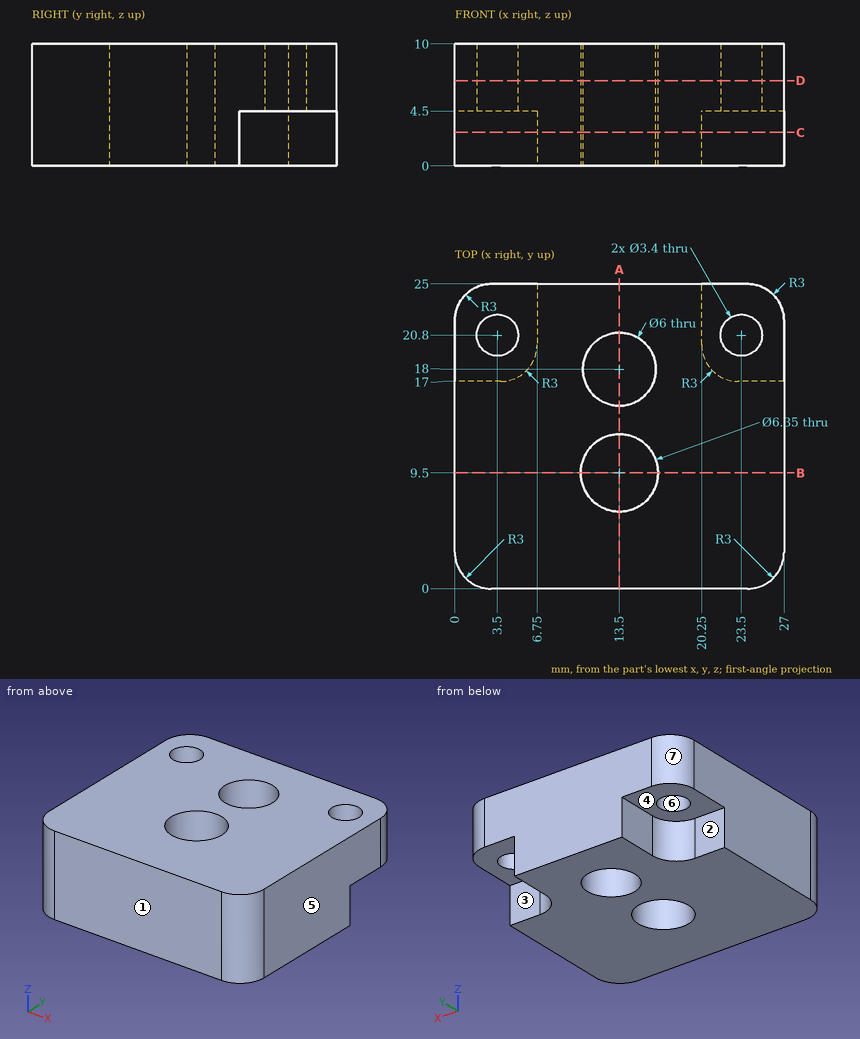
Could you check a few things on this drawing? It's one solid part, dimensions in mm from its lowest x, y, z. A direction names the side the tool comes from. Give positions to 0.01 mm unless a question says otherwise; leave off trailing zeros. Order: outer loops, then holes, each group sorted by start corner. A loop starts at its lowest first (then second) coordinate and runs counter-clockwise, first axis right, second up. Notation, with made-up numbers: (78.5, 54) - (110.5, 54) arc R7 cw to (110.5, 62) - close; hole circle Ø11 at (-3, 83). An arc over 180 degrees is marked (long way). One line per item, written item: value. Start each with the question number.
1. Imagine slicing it at D-D on z = 7. List the corners of the cut face in (x, y) for me (3 decimals).
2. If I drill on probe 1 along Y at (x, z) = (13.5, 5) (3 decimals); probe 2 along Y at (x, z) = (3.5, 6.3); probe 3 along X at (y, z) = (20.5, 8.75), over which ranges is the centre line in solid material (lowest first)?
3. For P1, Ø4.5, axis at x = 23.5, y = 20.8, coming from the -Z side; P2, Ø8, axis at x = 13.5, y = 18, coming from the +Z side; P3, Ø3, axis at x = 26, z = 1.5, coming from the +Y side; P4, Ø3.5, axis at y = 23, z = 2, coming from the +X side, each with a flat end and sliding along its axis, tell me the tip position at first contact or that it passes through.
4. Imagine slicing it at A-A on x = 13.5. List the corners of the cut face in (y, z) for me (3 decimals).
5. For the marked faces 1, 2 and 3, which set-ups out of +Z, -Z, +X, -X, +Y, -Y let a thin tool reach every point of the face, with its end or its side?
6. Thinking about a two-plate mould opening in X: for the marked faces 4, 5, 6 and 7, which applies, +X half, -X half, draft (parallel to the pull), parting line (faces both ways), or undercut?
7. Imagine slicing it at B-B on y = 9.5. List the corners of the cut face in (x, z) for me (3 decimals).
8. Imagine slicing it at C-C on z = 2.75. List the corners of the cut face in (x, y) for me (3 decimals).
Values:
1. outline: (0, 3) arc R3 ccw to (3, 0) - (24, 0) arc R3 ccw to (27, 3) - (27, 22) arc R3 ccw to (24, 25) - (3, 25) arc R3 ccw to (0, 22) - close; hole circle Ø3.4 at (3.5, 20.8); hole circle Ø6.35 at (13.5, 9.5); hole circle Ø6 at (13.5, 18); hole circle Ø3.4 at (23.5, 20.8)
2. probe 1: 0 to 6.325, 12.675 to 15, 21 to 25
2. probe 2: 0 to 19.1, 22.5 to 25
2. probe 3: 0 to 1.83, 5.17 to 11.84, 15.16 to 21.83, 25.17 to 27
3. P1: z = 4.5
3. P2: z = 10
3. P3: y = 17
3. P4: x = 20.25
4. outline: (0, 0) - (6.325, 0) - (6.325, 10) - (0, 10) - close; (12.675, 0) - (15, 0) - (15, 10) - (12.675, 10) - close; (21, 0) - (25, 0) - (25, 10) - (21, 10) - close
5. face 1: +Z, -Z, +X, -X, -Y
5. face 2: -Z, -X, +Y
5. face 3: -Z, +X, +Y
6. face 4: draft
6. face 5: +X half
6. face 6: undercut
6. face 7: -X half
7. outline: (0, 0) - (10.325, 0) - (10.325, 10) - (0, 10) - close; (16.675, 0) - (27, 0) - (27, 10) - (16.675, 10) - close
8. outline: (0, 3) arc R3 ccw to (3, 0) - (24, 0) arc R3 ccw to (27, 3) - (27, 17) - (23.25, 17) arc R3 cw to (20.25, 20) - (20.25, 25) - (6.75, 25) - (6.75, 20) arc R3 cw to (3.75, 17) - (0, 17) - close; hole circle Ø6.35 at (13.5, 9.5); hole circle Ø6 at (13.5, 18)
